The figure shows three views and two pictorial views of one solid part (mm, origin at its lowest corner). Answer the questions. A direction names the side the tool comes from. Coordinates: 2 decimals unless noted, no trailing zeros. Order: outer loops, then holes, each group sorted by start corner. A loop starts at its lowest first (then second) coordinate and runs counter-clockwise, first axis right, second up. Notation, with made-up numbers: (30.25, -22) -> (57.25, -22) arc R15 cw to (57.25, -16) -> close; hole circle Ø3 at (85, 72.5). An arc over 180 degrees is marked (long way). Use one line per item in the form item = value.
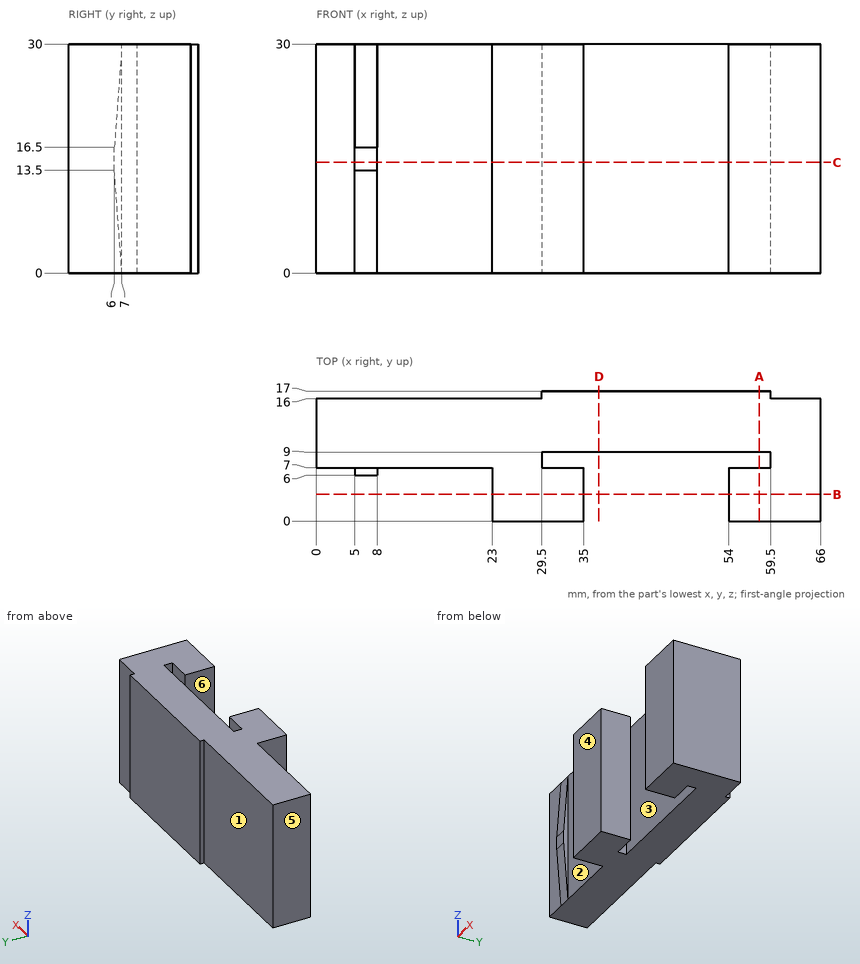
(1) Which of the six approach directions +Z, -Z, +X, -X, +Y, -Y give full straight-line access (tool end or side, diameter ignored) to the marked faces 1, 2 and 3?
Data:
face_1 = +Z, -Z, -X, +Y
face_2 = +Z, -Z, -Y
face_3 = +Z, -Z
(2) Straight lines are drawn through the part: line 1 along X through (y, z) = (1.75, 6.5); line 2 along Y through (x, z) = (31.5, 23); line 3 along Y through (x, z) = (42, 19). For each, find the intervals that lie inside material, in ascending order.
Data:
line_1 = 23 to 35, 54 to 66
line_2 = 0 to 7, 9 to 17
line_3 = 9 to 17
(3) Each of these flat-tipped pins is pushed along its axis until it touches: P1, Ø0.8, axis at y = 16.5, z = 13, coming from the +X side; P2, Ø9, axis at x = 15.5, z = 18, coming from the +Y side; P3, Ø1.1, axis at y = 16.5, z = 22, coming from the -X side; P4, Ø7.5, axis at x = 13.5, z = 18.5, coming from the -Y side. Where does it stop, or does it pass through?
Data:
P1 = 59.5
P2 = 16
P3 = 0
P4 = 7
(4) The mould has two halves that part along X. Classify the marked faces 4, 5 and 6: released by +X, released by -X, zero draft, split by the parting line, or undercut.
Data:
face_4 = zero draft
face_5 = released by -X
face_6 = undercut
(5) Section C-C on z = 14.5 is taken. Write down the section's boundary in (x, y).
Data:
outline = (0, 7) -> (5, 7) -> (5, 6) -> (8, 6) -> (8, 7) -> (23, 7) -> (23, 0) -> (35, 0) -> (35, 7) -> (29.5, 7) -> (29.5, 9) -> (59.5, 9) -> (59.5, 7) -> (54, 7) -> (54, 0) -> (66, 0) -> (66, 16) -> (59.5, 16) -> (59.5, 17) -> (29.5, 17) -> (29.5, 16) -> (0, 16) -> close
(6) Section B-B on y = 3.5 is taken. Write down the section's boundary in (x, z).
Data:
outline = (23, 0) -> (35, 0) -> (35, 30) -> (23, 30) -> close; (54, 0) -> (66, 0) -> (66, 30) -> (54, 30) -> close
(7) Section D-D on x = 37 is taken. Write down the section's boundary in (y, z).
Data:
outline = (9, 0) -> (17, 0) -> (17, 30) -> (9, 30) -> close
(8) Section A-A on x = 58 is taken. Write down the section's boundary in (y, z), plus the area to 3 significant figures.
Data:
outline = (0, 0) -> (7, 0) -> (7, 30) -> (0, 30) -> close; (9, 0) -> (17, 0) -> (17, 30) -> (9, 30) -> close
area = 450 mm²
